from build123d import *

# Parameters (mm, degrees)
EXTRUDE_1_DEPTH     = 10
SKETCH_2_R          = 28
SKETCH_2_R_2        = 22.5
EXTRUDE_2_DEPTH     = 8
SKETCH_3_R          = 32.5
SKETCH_3_R_2        = 29
EXTRUDE_3_DEPTH     = 40
SKETCH_4_R          = 32.5
EXTRUDE_4_DEPTH     = 11
RIB_4_REACH         = 112.057
SKETCH_5_WALL_W     = 291.205309728
SKETCH_5_WALL_H     = 8
SKETCH_6_W          = 24.014667972
SKETCH_6_H          = 9.139910945
CUT_EXTRUDE_1_DEPTH = 16


with BuildPart() as part:
    # Sketch 1 → Extrude 1 (new body)
    with BuildSketch(Plane.XY):
        with BuildLine():
            Line((0, 60), (-24, 60))
            Line((-24, 60), (-27.935985851, 1.892272326))
            ThreePointArc((-27.935985851, 1.892272326), (0, -28), (27.935985851, 1.892272326))
            Line((27.935985851, 1.892272326), (24, 60))
            Line((24, 60), (0, 60))
        make_face()
    extrude(amount=EXTRUDE_1_DEPTH)

    # Sketch 2 → Extrude 2 (add)
    with BuildSketch(Plane.XY.offset(10)):
        with Locations(Location((0, 0, 0), (0, 0, 176.124931535))):
            Circle(SKETCH_2_R)
        Circle(SKETCH_2_R_2, mode=Mode.SUBTRACT)
    extrude(amount=EXTRUDE_2_DEPTH)



with BuildPart() as body_2:
    # Sketch 3 → Extrude 3 (new body)
    with BuildSketch(Plane(origin=(0, 60, 0), x_dir=(1, 0, 0), z_dir=(0, 1, 0))):
        with Locations(Location((0, 0, 0), (0, 0, 270))):
            Circle(SKETCH_3_R)
        with Locations(Location((0, 0, 0), (0, 0, 270))):
            Circle(SKETCH_3_R_2, mode=Mode.SUBTRACT)
    extrude(amount=EXTRUDE_3_DEPTH)


with BuildPart() as part_1:
    add(part.part)

    add(body_2.part)  # Extrude 4 merges body 2
    # Sketch 4 → Extrude 4 (add)
    with BuildSketch(Plane.XZ.offset(-60)):
        with Locations(Location((0, 0, 0), (0, 0, 90))):
            Circle(SKETCH_4_R)
    extrude(amount=EXTRUDE_4_DEPTH)

    # Sketch 5 wall → Rib 4 (add, up to next)
    with BuildSketch(Plane(origin=(0, 16.604964226, -11.999062573), x_dir=(0, 0.937740264285, -0.347337295346), z_dir=(0, 0.347337295346, 0.937740264285)), mode=Mode.PRIVATE) as rib_4_sk1:
        Rectangle(SKETCH_5_WALL_W, SKETCH_5_WALL_H)
    rib_4_tool1 = extrude(rib_4_sk1.sketch, amount=RIB_4_REACH, mode=Mode.PRIVATE) - part_1.part
    add(rib_4_tool1.solids().sort_by_distance((0, 16.604964226, -11.999062573))[0])

    # Sketch 6 → Cut-Extrude 1 (cut)
    with BuildSketch(Plane(origin=(0, 60, 0), x_dir=(1, 0, 0), z_dir=(0, 1, 0))):
        with Locations((0, -21.281655386)):
            Rectangle(SKETCH_6_W, SKETCH_6_H)
    extrude(amount=-CUT_EXTRUDE_1_DEPTH, mode=Mode.SUBTRACT)


solid = part_1.part
The model under review builds one solid part; all positions refer to its coordinate system, in mm. A direction names the side the tool comes from. Give positions to 0.01 mm unless a question says otherwise; leave off trailing zeros. Write each loop counter-clockwise with the first axis right and the second up, starting at its lowest first coordinate (ties: lowest second). Pieces come first, ordered by that corner, then holes. Notation, with made-up numbers: M 0,37 L 26,37 A26 cw 26,68 Z; hole C -30,65.25 d4. An arc over 180 degrees is marked long. One line per question, with ' | ' between items. Start each with the question number.
Item 1: Wall thickness on line 1 (Y direction, x = 0, z = 13.75); line 2 (X direction, y = 73, z = 0); line 3 (Y direction, x = -17, z = -8): over which ranges is each line inside the solid? List them lowest first. Write a range as from..to.
Item 2: We need section D-D on y = 6. Write out the cut boundary in (x, z).
Item 3: We need section B-B on x = 0. Write out the cut boundary in (y, z).
Item 4: We need section A-A on z = 12.5. Write out the cut boundary in (x, y), plus the area to 3 significant figures.
Item 5: For faces 4 (the flat face through (6.8, 49, -0.5)), 5 (the flat face through (0, 55, 25.852)), 6 (the flat face through (4, 25, -9)), 7 (the flat face through (0, 0, 10)), list the 3-axis set-ups (+Z, -Z, +X, -X, +Y, -Y) from which the entire face can be reached by the end or side of a thin tool; tool diameter is ignored.
Item 6: We need section C-C on z = 20. Write out the cut boundary in (x, y).
Item 7: Draft analysis for pull direction Y (two halves, no side actions). For faces 1 (the flat face through (26.363, 25.116, 4.93)), 2 (the flat face through (-0.06, 16.15, -11.83)), 3 (the flat face through (6, 11, 0)), state which applies: released by +Y, released by -Y, zero draft, split by the parting line, or undercut.
Item 8: For pin 1 (8 mm diameter, centred on x = -21, z = 24, fed in from -Y); pin 2 (10 mm diameter, centred on y = 53, z = 22, fed in from +X); pin 3 (14 mm diameter, centred on x = -7.5, y = 23.5, fed in from +Z), all flat-tipped, find the tip position at first contact; note any pin that passes through.
Results found:
1) line 1: y = -28..-22.5, 22.5..28, 49..60 | line 2: x = -32.5..-29, 29..32.5 | line 3: y = 49..60
2) outline: M -27.66,0 L -4,0 L -4,-8.07 L 4,-8.07 L 4,0 L 27.66,0 L 27.66,10 L 27.35,10 L 27.35,18 L 21.69,18 L 21.69,10 L -21.69,10 L -21.69,18 L -27.35,18 L -27.35,10 L -27.66,10 Z
3) outline: M -28,0 L -15.79,0 L 49,-24 L 49,-32.5 L 100,-32.5 L 100,-29 L 60,-29 L 60,16.71 L 49,16.71 L 49,10 L 28,10 L 28,18 L 22.5,18 L 22.5,10 L -22.5,10 L -22.5,18 L -28,18 Z; M 49,25.85 L 60,25.85 L 60,29 L 100,29 L 100,32.5 L 49,32.5 Z
4) outline: M -30,49 L 30,49 L 30,100 L 26.17,100 L 26.17,60 L -26.17,60 L -26.17,100 L -30,100 Z; C 0,0 d56; hole C 0,0 d45 | area: 1,840 mm2
5) face 4: none | face 5: +Y, -Y | face 6: -Z, +X, -Y | face 7: +Z
6) outline: M -25.62,49 L -12.01,49 L -12.01,60 L -21,60 L -21,100 L -25.62,100 Z; M 12.01,49 L 25.62,49 L 25.62,100 L 21,100 L 21,60 L 12.01,60 Z
7) face 1: undercut | face 2: released by -Y | face 3: zero draft
8) pin 1: stops at y = 49 | pin 2: stops at x = 27.7 | pin 3: stops at z = 18
